from build123d import *

# Parameters (mm, degrees)
BOSS_EXTRUDE1_DEPTH = 10
BOSS_EXTRUDE2_DEPTH = 65
SKETCH5_R           = 2.7
M5HOLES_DEPTH       = 231.341689519
SKETCH6_R           = 2.7
M5_HOLES_DEPTH      = 25
SKETCH7_W           = 7.5
SKETCH7_H           = 15
BOSS_EXTRUDE3_DEPTH = 121


with BuildPart() as part:
    # Sketch1 → Boss-Extrude1 (new body)
    with BuildSketch(Plane(origin=(0, 0, 0), x_dir=(1, 0, 0), z_dir=(0, 1, 0))):
        Polygon((-142.5, 141.171435272), (-142.5, 152.421435272), (-162.5, 152.421435272), (-162.5, 32.421435272), (-2.5, 32.421435272), (-2.5, 152.421435272), (-22.5, 152.421435272), (-22.5, 141.171435272), (-17.5, 141.171435272), (-17.5, 43.671435272), (-147.5, 43.671435272), (-147.5, 141.171435272), align=None)
    extrude(amount=BOSS_EXTRUDE1_DEPTH)

    # Sketch2 → Boss-Extrude2 (add)
    with BuildSketch(Plane.XZ):
        Polygon((-156, -144.921435272), (-156, -39.921435272), (-9, -39.921435272), (-9, -144.921435272), (-22.5, -144.921435272), (-22.5, -152.421435272), (-2.5, -152.421435272), (-2.5, -32.421435272), (-162.5, -32.421435272), (-162.5, -152.421435272), (-142.5, -152.421435272), (-142.5, -144.921435272), align=None)
    extrude(amount=BOSS_EXTRUDE2_DEPTH)

    # Sketch5 → M5holes (cut, through all)
    with BuildSketch(Plane.ZY.offset(162.5)):
        with Locations((-132.421435272, -57.5)):
            Circle(SKETCH5_R)
        with Locations((-112.421435272, -57.5)):
            Circle(SKETCH5_R)
        with Locations((-92.421435272, -57.5)):
            Circle(SKETCH5_R)
        with Locations((-72.421435272, -57.5)):
            Circle(SKETCH5_R)
        with Locations((-52.421435272, -57.5)):
            Circle(SKETCH5_R)
    extrude(amount=-M5HOLES_DEPTH, mode=Mode.SUBTRACT)

    # Sketch6 → M5_holes (cut)
    with BuildSketch(Plane(origin=(0, 0, -39.921435272), x_dir=(-1, 0, 0), z_dir=(0, 0, -1))):
        with Locations((29, -57.5)):
            Circle(SKETCH6_R)
        with Locations((54, -57.5)):
            Circle(SKETCH6_R)
        with Locations((79, -57.5)):
            Circle(SKETCH6_R)
        with Locations((104, -57.5)):
            Circle(SKETCH6_R)
        with Locations((129, -57.5)):
            Circle(SKETCH6_R)
    extrude(amount=-M5_HOLES_DEPTH, mode=Mode.SUBTRACT)

    # Sketch7 → Boss-Extrude3 (add)
    with BuildSketch(Plane.ZY.offset(22.5)):
        with Locations((-148.671435272, -57.5)):
            Rectangle(SKETCH7_W, SKETCH7_H)
    extrude(amount=BOSS_EXTRUDE3_DEPTH)


solid = part.part
Here's how the part is built. I have some questions about the finished solid (model axes, mm). A direction names the side the tool comes from. Coordinates: 2 decimals unless noted, no trailing zeros. Loops run counter-clockwise (first coordinate to the right, second up) from the corner with the lowest first, then second, coordinate; pieces in that order, holes last.
1. For P1, Ø1.5, axis at x = -52, y = -32, coming from the -Z side, with a flat end and sliding along its axis, tell me the tip position at first contact or that it passes through.
2. Imagine slicing it at D-D, the plane x = -29. Please give me the cut outline in (y, z), and give its area (3 significant figures).
3. Imagine slicing it at A-A, the plane z = -88. Please give me the cut outline in (x, y).
4. For faces 1 (the flat face through (-147.5, 5, -92)), 2 (the cylindrical face through (-130.246, -59.895, -36.224)), 3 (the flat face through (-99, 0, -42)), 4 (the flat face through (-142.5, -20, -148)), which set-ups out of +Z, -Z, +X, -X, +Y, -Y let a thin tool reach every point of the face, with its end or its side?
5. Imagine slicing it at C-C, the plane y = -31. Please give me the cut outline in (x, z), and give its area (4 significant figures).
6. Imagine slicing it at B-B, the plane x = -117. Please give me the cut outline in (y, z).
7. If we mould it in two halves opening along X, with no side actions, what happens to faces 5 (the cylindrical face through (-159.296, -60.136, -113.007)), 6 (the flat face through (-9, -32, -92)), 7 (the flat face through (-84, -32, -39.921))? For each: pulls with the +X half, pulls with the -X half, needs draft (parallel to the pull), parting line crosses it, or undercut.
8. I need wall thicknesses on L1, parallel to Z at x = -14, y = -2; L2, parallel to X at y = -17, z = -134.5; L3, parallel to Z at x = -6, y = -57. Which ranges of each line are inside material? Lowest first, please.
Taken from the geometry:
1. P1: stops at z = -39.92
2. outline: (-65, -152.42) - (-50, -152.42) - (-50, -144.92) - (-65, -144.92) - close; (-65, -39.92) - (-60.2, -39.92) - (-60.2, -32.42) - (-65, -32.42) - close; (-54.8, -39.92) - (0, -39.92) - (0, -43.67) - (10, -43.67) - (10, -32.42) - (-54.8, -32.42) - close
2. area: 672 mm2
3. outline: (-162.5, -65) - (-156, -65) - (-156, 0) - (-147.5, 0) - (-147.5, 10) - (-162.5, 10) - close; (-17.5, 0) - (-9, 0) - (-9, -65) - (-2.5, -65) - (-2.5, 10) - (-17.5, 10) - close
4. face 1: +Y, -Y
4. face 2: +Z
4. face 3: -Y
4. face 4: -Z, +Y
5. outline: (-162.5, -152.42) - (-142.5, -152.42) - (-142.5, -144.92) - (-156, -144.92) - (-156, -39.92) - (-9, -39.92) - (-9, -144.92) - (-22.5, -144.92) - (-22.5, -152.42) - (-2.5, -152.42) - (-2.5, -32.42) - (-162.5, -32.42) - close
5. area: 2,865 mm2
6. outline: (-65, -152.42) - (-50, -152.42) - (-50, -144.92) - (-65, -144.92) - close; (-65, -39.92) - (0, -39.92) - (0, -43.67) - (10, -43.67) - (10, -32.42) - (-65, -32.42) - close
7. face 5: needs draft
7. face 6: undercut
7. face 7: undercut
8. L1: z = -152.42 to -144.92, -39.92 to -32.42
8. L2: x = -162.5 to -156, -9 to -2.5
8. L3: z = -152.42 to -135.07, -129.77 to -115.07, -109.77 to -95.07, -89.77 to -75.07, -69.77 to -55.07, -49.77 to -32.42
